from build123d import *

# Parameters (mm, degrees)
SKETCH_1_R          = 2.65
EXTRUDE_1_DEPTH     = 20
CUT_EXTRUDE_1_DEPTH = 10
FILLET_1_R          = 2
FILLET_2_R          = 30
SKETCH_3_R          = 1.65
CUT_EXTRUDE_2_DEPTH = 58.468525672
FILLET_3_R          = 6


with BuildPart() as part:
    # 草图1 → 凸台-拉伸1 (new body)
    with BuildSketch(Plane.XY):
        with BuildLine():
            Line((0, 0), (0, 13))
            ThreePointArc((0, 13), (7.89575828, 24.276311449), (21.192533317, 20.713451316))
            Line((21.192533317, 20.713451316), (35.365655494, 3.822582044))
            Line((35.365655494, 3.822582044), (35.365655494, -31.177417956))
            ThreePointArc((35.365655494, -31.177417956), (35.245743493, -40.47423292), (34.886087273, -49.764862326))
            ThreePointArc((34.886087273, -49.764862326), (26.594605872, -36.149168843), (15.158760375, -25.042539714))
            Line((15.158760375, -25.042539714), (10.158760375, -16.382285677))
            Line((10.158760375, -16.382285677), (14.488887394, -13.882285677))
            Line((14.488887394, -13.882285677), (14.488887394, -3.882285677))
            Line((14.488887394, -3.882285677), (0, 0))
        make_face()
        with Locations((12, 13)):
            Circle(SKETCH_1_R, mode=Mode.SUBTRACT)
    extrude(amount=EXTRUDE_1_DEPTH)

    # 草图2 → 切除-拉伸1 (cut)
    with BuildSketch(Plane.XY.offset(20)):
        Polygon((15.158760375, -25.042539714), (35.365655494, -7.132145445), (35.365655494, -70.887668239), (13.758782183, -70.887668239), align=None)
    extrude(amount=-CUT_EXTRUDE_1_DEPTH, mode=Mode.SUBTRACT)

    # 圆角1
    fillet_1_edges = [part.edges().sort_by_distance(p)[0] for p in [
        (34.886087273, -49.764862326, 5),
    ]]
    fillet(fillet_1_edges, radius=FILLET_1_R)

    # 圆角2
    fillet_2_edges = [part.edges().sort_by_distance(p)[0] for p in [
        (35.365655494, 3.822582044, 10),
    ]]
    fillet(fillet_2_edges, radius=FILLET_2_R)

    # 草图3 → 切除-拉伸2 (cut, through all)
    with BuildSketch(Plane.XY.offset(10)):
        with Locations((25.95004871, -26.58161927)):
            Circle(SKETCH_3_R)
    extrude(amount=-CUT_EXTRUDE_2_DEPTH, mode=Mode.SUBTRACT)

    # 圆角3
    fillet_3_edges = [part.edges().sort_by_distance(p)[0] for p in [
        (0, 0, 10),
    ]]
    fillet(fillet_3_edges, radius=FILLET_3_R)


solid = part.part
Here's how the part is built. I have some questions about the finished solid (model axes, mm). A direction names the side the tool comes from. Round coordinates to 2 decimals unless told otherwise and drop trailing zeros. Loops run counter-clockwise (first coordinate to the right, second up) from the corner with the lowest first, then second, coordinate; pieces in that order, holes last. Notation, with made-up numbers: M 63.25,13 L 97.25,13 A14 ccw 97.25,21 Z; hole C -12,32.25 d6. An arc over 180 degrees is marked long. Write each question's results on one line, items separated by ' | '. Start each with the question number.
(1) Will these pins go through, and if not, where does the flat tip stop? P1, Ø6, axis at x = 12, y = 13, coming from the -Z side; P2, Ø8, axis at x = 28.5, z = 3, coming from the -Y side; P3, Ø11, axis at y = -10.5, z = 14.5, coming from the -X side; P4, Ø5, axis at x = 7.5, y = -15, coming from the +Z side.
(2) On a 3-axis mill with a long thin cutter (end or side, diameter ignored), from which of +Z, -Z, +X, -X, +Y, -Y can I reach the whole of each face in a straight line? I mean faces 1 (the flat face through (14.489, -9, 10)), 2 (the cylindrical face through (35.324, -36.633, 4.93)), 3 (the cylindrical face through (7.703, 24.204, 9.86)), 4 (the flat face through (12.69, -20.77, 9.86)), 5 (the flat face through (25.121, -16.213, 15.07)). Say none if no direction works.
(3) I want a section at C-C (y = 6). Please give me the cut outline in (x, z), then the cut area to 3 significant figures.
(4) If I drill on probe 1 along Z at (x, y) = (28, -23.5); probe 2 along Y at (x, z) = (25, 7.25); probe 3 along Y at (x, z) = (5, 9), over which ranges is the centre line in solid material (lowest first)? Write a range as from..to.
(5) I want a section at D-D (z = 7.5). State how many separate pieces and enclosed holes the cut face has, then the cut area to 3 significant figures.
(6) I want a section at A-A (x = 13.5). Please give me the cut outline in (y, z).
(7) Thinking about a two-plate mould opening in X: for faces 6 (the flat face through (18, 0, 20)), 7 (the flat face through (35.366, -19, 5)), 8 (the cylindrical face through (13.223, 10.649, 9.86)), 9 (the cylindrical face through (24.319, -33.456, 4.93)), which applies, pulls with the +X half, pulls with the -X half, needs draft (parallel to the pull), parting line crosses it, or undercut?
Solved:
1) P1: stops at z = 0 | P2: stops at y = -44.06 | P3: stops at x = 10.82 | P4: passes through
2) face 1: +Z, -Z, -X | face 2: +Z, -Z, +X, -Y | face 3: +Z, -Z, +Y | face 4: +Z, -Z, -X, -Y | face 5: +Z, +X, -Y
3) outline: M 0,0 L 32.36,0 L 32.36,20 L 0,20 Z | area: 647 mm²
4) probe 1: z = 0..10 | probe 2: y = -34.23..-27.93, -25.23..16.18 | probe 3: y = -1.34..22.75
5) separate pieces: 1 | enclosed holes: 2 | area: 1,390 mm²
6) outline: M -22.17,0 L -14.45,0 L -14.45,20 L -22.17,20 Z; M -3.62,0 L 10.82,0 L 10.82,20 L -3.62,20 Z; M 15.18,0 L 24.91,0 L 24.91,20 L 15.18,20 Z
7) face 6: needs draft | face 7: pulls with the +X half | face 8: undercut | face 9: pulls with the -X half
